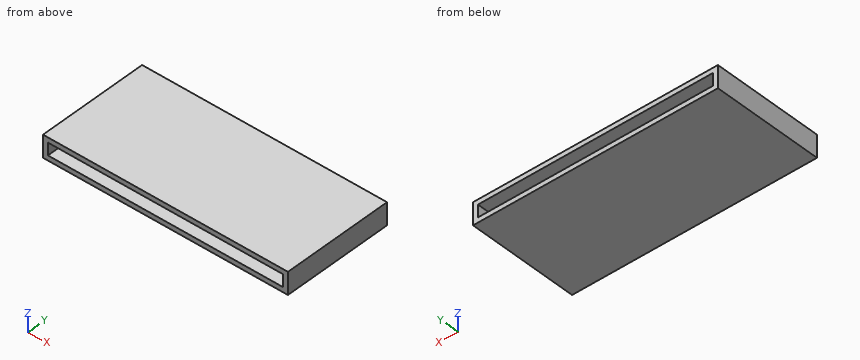
```python
from build123d import *

# Parameters (mm, degrees)
SKETCH1_W           = 198.621366483
SKETCH1_H           = 90
BOSS_EXTRUDE1_DEPTH = 4
SKETCH3_W           = 4
SKETCH3_H           = 90
BOSS_EXTRUDE2_DEPTH = 10
SKETCH21_W          = 198.621366483
SKETCH21_H          = 90
BOSS_EXTRUDE3_DEPTH = 4


with BuildPart() as part:
    # Sketch1 → Boss-Extrude1 (new body)
    with BuildSketch(Plane.XY):
        with Locations((99.310683242, 45)):
            Rectangle(SKETCH1_W, SKETCH1_H)
    extrude(amount=BOSS_EXTRUDE1_DEPTH)

    # Sketch3 → Boss-Extrude2 (add)
    with BuildSketch(Plane.XY.offset(4)):
        with Locations((2, 45)):
            Rectangle(SKETCH3_W, SKETCH3_H)
        with Locations((196.621366483, 45)):
            Rectangle(SKETCH3_W, SKETCH3_H)
    extrude(amount=BOSS_EXTRUDE2_DEPTH)

    # Sketch21 → Boss-Extrude3 (add)
    with BuildSketch(Plane.XY.offset(14)):
        with Locations((99.310683242, 45)):
            Rectangle(SKETCH21_W, SKETCH21_H)
    extrude(amount=BOSS_EXTRUDE3_DEPTH)


solid = part.part
```
For this review, take the finished solid that the model builds, in its own axes (mm). Coordinates: 2 decimals unless noted, no trailing zeros. Loops run counter-clockwise (first coordinate to the right, second up) from the corner with the lowest first, then second, coordinate; pieces in that order, holes last.
1. For line 1 (Z direction, x = 130, y = 38); line 2 (X direction, y = 74, z = 5.75), list the stretches that pass through material, from the lowest coordinate up.
2. Add section A-A, the plane y = 31. Give the boundary of the cut face in (x, z), then the cut area to 3 significant figures.
3. Insertion check: P1, Ø8, axis at x = 131.5, z = 12, coming from the +Y side. The pin has a flat end and moves straight along its axis. Give the tip position at first contact, or say it passes through.
4. Add section B-B, the plane z = 6.5. Give the boundary of the cut face in (x, y).
5. Add section C-C, the plane x = 110. Give the boundary of the cut face in (y, z), then the cut area to 3 significant figures.
Result:
1. line 1: z = 0 to 4, 14 to 18
1. line 2: x = 0 to 4, 194.62 to 198.62
2. outline: (0, 0) - (198.62, 0) - (198.62, 18) - (0, 18) - close; hole (4, 4) - (194.62, 4) - (194.62, 14) - (4, 14) - close
2. area: 1,670 mm2
3. P1: stops at y = 90
4. outline: (0, 0) - (4, 0) - (4, 90) - (0, 90) - close; (194.62, 0) - (198.62, 0) - (198.62, 90) - (194.62, 90) - close
5. outline: (0, 0) - (90, 0) - (90, 4) - (0, 4) - close; (0, 14) - (90, 14) - (90, 18) - (0, 18) - close
5. area: 720 mm2
